The model under review builds one solid part; all positions refer to its coordinate system, in mm. Face numbers are marked on the shaded views. A direction names the side the tool comes from. Round coordinates to 2 decimals unless told otherwise and drop trailing zeros. Loops run counter-clockwise (first coordinate to the right, second up) from the corner with the lowest first, then second, coordinate; pieces in that order, holes last. Notation, with made-up numbers: M 56,57.5 L 110,57.5 A33 cw 110,94.5 Z; hole C 1.25,-9.5 d10. An arc over 180 degrees is marked long. Return JSON: item names as keys, results as strings. Group by question number.
Q1. Consider section D-D (x = 14.25). State the section outline as (y, z) points.
Q2. Clearance check with a flat-ended pin moving along its axis: pin 1 Ø3 at (x, z) = (10, 21.25) entering from -Y. State where the tip first meets the part, or that it passes through.
Q3. For the marked faces 1 and 2, list the 3-axis set-ups (+Z, -Z, +X, -X, +Y, -Y) from which the entire face can be reached by the end or side of a thin tool; tool diameter is ignored.
Q4. Draft analysis for pull direction Y (two halves, no side actions). For the marked faces 3, 4 and 5, state which applies: pulls with the +Y half, pulls with the -Y half, needs draft (parallel to the pull), parting line crosses it, or undercut.
Q5. Consider section A-A (z = 21.25). State the section outline as (x, y) points, and give its area (3 significant figures).
Q6. Consider section C-C (y = 11.5). State the section outline as (x, z) points, and give its area (3 significant figures).
Q7. Consider section B-B (x = 10). State the section outline as (y, z) points, and give its area (3 significant figures).
Q8. To check wall thickness, follow line 1 along Z through (x, y) = (10, -14.3); line 2 along Z through (x, y) = (12, 3.5); line 3 along X through (y, z) = (-14.4, 21.25). State the ranges of each line that lie inside material, in increasing order.
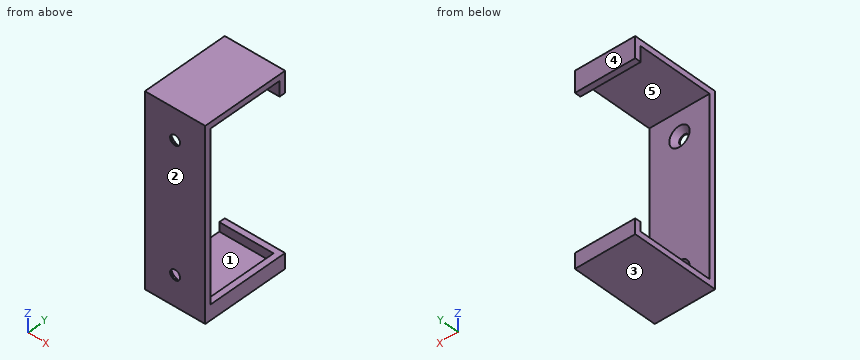
from build123d import *

# Parameters (mm, degrees)
F0_W           = 29
F0_H           = 62.5
F0_W_2         = 25
F0_H_2         = 58.5
F1_DEPTH       = 20
F2_W           = 20
F2_H           = 52.5
F3_DEPTH       = 2
F5_D           = 3.3
F5_CSINK_D     = 6.72
F5_CSINK_ANGLE = 90
F6_W           = 2
F6_H           = 25
F7_DEPTH       = 3
F8_DEPTH       = 2


with BuildPart() as f1:
    # F0 (on Right) → F1 (new body)
    with BuildSketch(Plane.YZ):
        Rectangle(F0_W, F0_H)
        Rectangle(F0_W_2, F0_H_2, mode=Mode.SUBTRACT)
    extrude(amount=F1_DEPTH)

    # F2 (on face) → F3 (cut)
    with BuildSketch(Plane(origin=(0, 14.5, 0), x_dir=(-1, 0, 0), z_dir=(0, 1, 0))):
        with Locations((-10, 0)):
            Rectangle(F2_W, F2_H)
    extrude(amount=-F3_DEPTH, mode=Mode.SUBTRACT)

    # F5 (through all)
    with Locations(Plane(origin=(0, -12.5, 0), x_dir=(-1, 0, 0), z_dir=(0, 1, 0))):
        with Locations((-10, 21.25), (-10, -21.25)):
            CounterSinkHole(F5_D / 2, F5_CSINK_D / 2, counter_sink_angle=F5_CSINK_ANGLE)

    # F6 (on face) → F7 (join, through all)
    with BuildSketch(Plane.XY.offset(-29.25)):
        with Locations((19, 0)):
            Rectangle(F6_W, F6_H)
    extrude(amount=F7_DEPTH)

    # F8 (add): a face of the model
    f8_faces = [f1.faces().sort_by_distance(p)[0] for p in [
        (10, 13.5, 26.25),
    ]]
    extrude(f8_faces, amount=F8_DEPTH)


solid = f1.part
Values:
{
 "1": {"outline": "M -14.5,-31.25 L 14.5,-31.25 L 14.5,-26.25 L 12.5,-26.25 L 12.5,-29.25 L -12.5,-29.25 L -12.5,29.25 L 12.5,29.25 L 12.5,24.25 L 14.5,24.25 L 14.5,31.25 L -14.5,31.25 Z"},
 "2": {"pin 1": "passes through"},
 "3": {"face 1": "-X", "face 2": "+Z, -Z, +X, -X, -Y"},
 "4": {"face 3": "needs draft", "face 4": "pulls with the +Y half", "face 5": "undercut"},
 "5": {"outline": "M 0,-14.5 L 8.35,-14.5 L 8.35,-14.21 L 6.64,-12.5 L 0,-12.5 Z; M 11.65,-14.5 L 20,-14.5 L 20,-12.5 L 13.36,-12.5 L 11.65,-14.21 Z", "area": "30.5 mm2"},
 "6": {"outline": "M 0,-31.25 L 20,-31.25 L 20,-26.25 L 18,-26.25 L 18,-29.25 L 0,-29.25 Z; M 0,29.25 L 20,29.25 L 20,31.25 L 0,31.25 Z", "area": "86.0 mm2"},
 "7": {"outline": "M -14.5,-31.25 L 14.5,-31.25 L 14.5,-26.25 L 12.5,-26.25 L 12.5,-29.25 L -12.5,-29.25 L -12.5,-24.61 L -14.21,-22.9 L -14.5,-22.9 Z; M -14.5,-19.6 L -14.21,-19.6 L -12.5,-17.89 L -12.5,17.89 L -14.21,19.6 L -14.5,19.6 Z; M -14.5,22.9 L -14.21,22.9 L -12.5,24.61 L -12.5,29.25 L 12.5,29.25 L 12.5,24.25 L 14.5,24.25 L 14.5,31.25 L -14.5,31.25 Z", "area": "230 mm2"},
 "8": {"line 1": "z = -31.25 to -22.9, -19.6 to 19.6, 22.9 to 31.25", "line 2": "z = -31.25 to -29.25, 29.25 to 31.25", "line 3": "x = 0 to 8.35, 11.65 to 20"}
}
